```python
from build123d import *

# Parameters (mm, degrees)
SKETCH1_R           = 5
BOSS_EXTRUDE1_DEPTH = 10
SKETCH2_R           = 3.25
CUT_EXTRUDE1_DEPTH  = 8
SKETCH3_R           = 1.25
BOSS_EXTRUDE2_DEPTH = 6
DOME1_FACE_RADIUS   = 1.25
DOME1_HEIGHT        = 1


with BuildPart() as part:
    # Sketch1 → Boss-Extrude1 (new body)
    with BuildSketch(Plane(origin=(0, 0, 0), x_dir=(1, 0, 0), z_dir=(0, 1, 0))):
        Circle(SKETCH1_R)
    extrude(amount=BOSS_EXTRUDE1_DEPTH)

    # Sketch2 → Cut-Extrude1 (cut)
    with BuildSketch(Plane(origin=(0, 10, 0), x_dir=(1, 0, 0), z_dir=(0, 1, 0))):
        Circle(SKETCH2_R)
    extrude(amount=-CUT_EXTRUDE1_DEPTH, mode=Mode.SUBTRACT)

    # Sketch3 → Boss-Extrude2 (add)
    with BuildSketch(Plane(origin=(0, 2, 0), x_dir=(1, 0, 0), z_dir=(0, 1, 0))):
        Circle(SKETCH3_R)
    extrude(amount=BOSS_EXTRUDE2_DEPTH)

    # Dome1: a dome of height H over a round flat face of radius A is a cap of a sphere of radius (A * A + H * H) / (2 * H)
    dome1_r = (DOME1_FACE_RADIUS * DOME1_FACE_RADIUS + DOME1_HEIGHT * DOME1_HEIGHT) / (2 * DOME1_HEIGHT)
    dome1_base = Plane((0, 8, 0), z_dir=(0, 1, 0))
    with Locations(dome1_base.offset(DOME1_HEIGHT - dome1_r)):
        dome1_ball = Sphere(dome1_r, mode=Mode.PRIVATE)
    add(split(dome1_ball, bisect_by=dome1_base, keep=Keep.TOP, mode=Mode.PRIVATE))


solid = part.part
```
Could you check a few things on this model? Use its own coordinates, in mm. A direction names the side the tool comes from. Coordinates: 2 decimals unless noted, no trailing zeros. Write each loop counter-clockwise with the first axis right and the second up, starting at its lowest first coordinate (ties: lowest second). Pieces come first, ordered by that corner, then holes. Notation, with made-up numbers: M 63.5,22.5 L 118.5,22.5 A17 ccw 118.5,28.5 Z; hole C 24.5,53.25 d10. An arc over 180 degrees is marked long. Answer as CSV lines item,"result". Start each with the question number.
1) We'd pull the mould along X, two halves only. Please class faces 1 (the flat face through (1.4, 2, -0.05)), 2 (the flat face through (0, 0, 0)), 3 (the cylindrical face through (-1.08, 4.93, 4.88)): +X half, -X half, draft (parallel to the pull), parting line (faces both ways), or undercut.
2) For faces 4 (the flat face through (1, 10, 3.3)), 5 (the cylindrical face through (-2.579, 6.056, 1.978)), which set-ups out of +Z, -Z, +X, -X, +Y, -Y let a thin tool reach every point of the face, with its end or its side?
3) I want a section at A-A, the plane y = 2.25. Please give me the cut outline in (x, z).
4) I want a section at D-D, the plane y = 9.75. Please give me the cut outline in (x, z), and give its area (3 significant figures).
5) I want a section at B-B, the plane z = 0. Please give me the cut outline in (x, y), and give its area (3 significant figures).
6) For P1, Ø4, axis at y = 4, z = -3.5, coming from the +X side; P2, Ø3, axis at x = 1, z = -1, coming from the +Y side; P3, Ø3, axis at x = -3.5, y = 5, coming from the -Z side, each with a flat end and sliding along its axis, tell me the tip position at first contact or that it passes through.
7) Please list where these lines run through material, in increasing order: line 1 (Z direction, x = 0, y = 5); line 2 (X direction, y = 5.5, z = 0.75). Write a range as from..to.
8) I want a section at C-C, the plane x = 2.75. Please give me the cut outline in (y, z).
Data:
1,face 1,"undercut"
1,face 2,"draft"
1,face 3,"parting line"
2,face 4,"+Z, -Z, +X, -X, +Y"
2,face 5,"+Y"
3,outline,"C 0,0 d10; C 0,0 d2.5; hole C 0,0 d6.5"
4,outline,"C 0,0 d10; hole C 0,0 d6.5"
4,area,"45.4 mm^2"
5,outline,"M -5,0 L 5,0 L 5,10 L 3.25,10 L 3.25,2 L 1.25,2 L 1.25,8 A1.28 ccw -1.25,8 L -1.25,2 L -3.25,2 L -3.25,10 L -5,10 Z"
5,area,"64.9 mm^2"
6,P1,"stops at x = 4.77"
6,P2,"stops at y = 9"
6,P3,"stops at z = -4.58"
7,line 1,"z = -5..-3.25, -1.25..1.25, 3.25..5"
7,line 2,"x = -4.94..-3.16, -1..1, 3.16..4.94"
8,outline,"M 0,-4.18 L 10,-4.18 L 10,-1.73 L 2,-1.73 L 2,1.73 L 10,1.73 L 10,4.18 L 0,4.18 Z"
